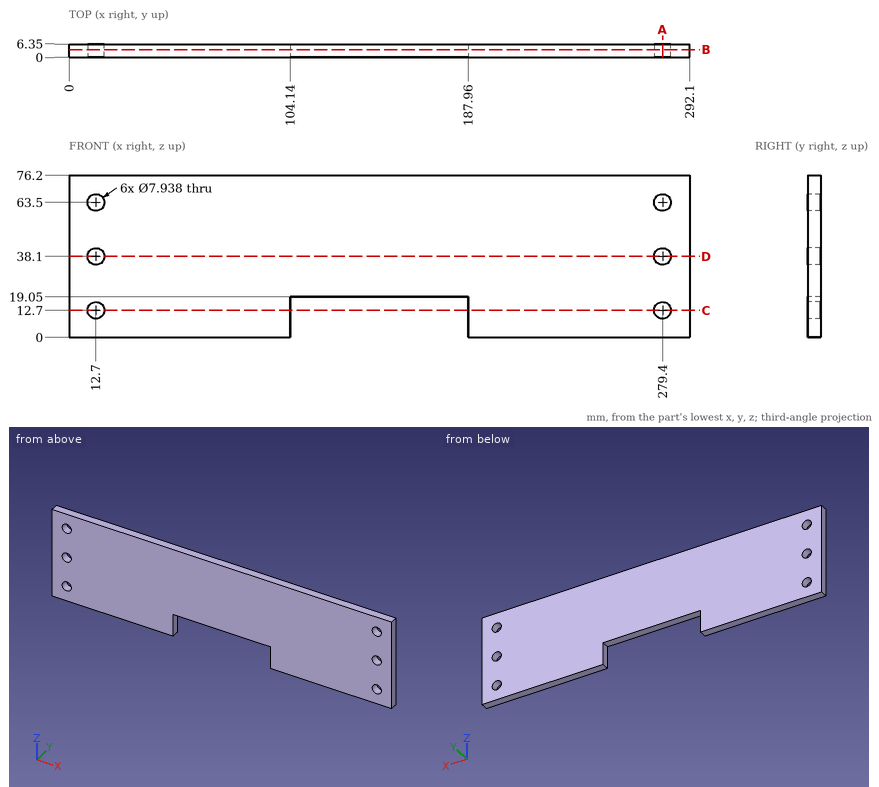
For this review, use the dimensioned drawing (mm, ordinates from the lowest corner) and the shaded views. Round coordinates to 2 decimals unless told otherwise and drop trailing zeros. Write each loop counter-clockwise with the first axis right and the second up, starting at its lowest first coordinate (ties: lowest second). Pieces come first, ordered by that corner, then holes. Notation, with made-up numbers: (73, 33.5) -> (92, 33.5) arc R15 ccw to (92, 61.5) -> close; hole circle Ø8 at (-30, 12.5). An arc over 180 degrees is marked (long way). Answer in a Markdown table with one row per item.
Q1. Take a section at B-B, the plane y = 3.75. State the section outline as (x, z) points.
The answers:
| item | result |
|---|---|
| outline | (0, 0) -> (104.14, 0) -> (104.14, 19.05) -> (187.96, 19.05) -> (187.96, 0) -> (292.1, 0) -> (292.1, 76.2) -> (0, 76.2) -> close; hole circle Ø7.94 at (12.7, 12.7); hole circle Ø7.94 at (12.7, 38.1); hole circle Ø7.94 at (12.7, 63.5); hole circle Ø7.94 at (279.4, 12.7); hole circle Ø7.94 at (279.4, 38.1); hole circle Ø7.94 at (279.4, 63.5) |
Q2. Take a section at C-C, the plane z = 12.7. State the section outline as (x, y) points.
The answers:
| item | result |
|---|---|
| outline | (0, 0) -> (8.73, 0) -> (8.73, 6.35) -> (0, 6.35) -> close; (16.67, 0) -> (104.14, 0) -> (104.14, 6.35) -> (16.67, 6.35) -> close; (187.96, 0) -> (275.43, 0) -> (275.43, 6.35) -> (187.96, 6.35) -> close; (283.37, 0) -> (292.1, 0) -> (292.1, 6.35) -> (283.37, 6.35) -> close |
Q3. Take a section at A-A, the plane x = 279.4. State the section outline as (y, z) points.
The answers:
| item | result |
|---|---|
| outline | (0, 0) -> (6.35, 0) -> (6.35, 8.73) -> (0, 8.73) -> close; (0, 16.67) -> (6.35, 16.67) -> (6.35, 34.13) -> (0, 34.13) -> close; (0, 42.07) -> (6.35, 42.07) -> (6.35, 59.53) -> (0, 59.53) -> close; (0, 67.47) -> (6.35, 67.47) -> (6.35, 76.2) -> (0, 76.2) -> close |
Q4. Clearance check with a flat-ended pin moving along its axis: pin 1 Ø5 at (x, z) = (12.7, 63.5) entering from -Y. State where the tip first meets the part, or that it passes through.
The answers:
| item | result |
|---|---|
| pin 1 | through |
Q5. Take a section at D-D, the plane z = 38.1. State the section outline as (x, y) points, then the cut area to 3 significant figures.
The answers:
| item | result |
|---|---|
| outline | (0, 0) -> (8.73, 0) -> (8.73, 6.35) -> (0, 6.35) -> close; (16.67, 0) -> (275.43, 0) -> (275.43, 6.35) -> (16.67, 6.35) -> close; (283.37, 0) -> (292.1, 0) -> (292.1, 6.35) -> (283.37, 6.35) -> close |
| area | 1,750 mm² |
Q6. To check wall thickness, follow L1, parallel to Z at x = 12.7, y = 2; L2, parallel to X at y = 3.75, z = 38.1; L3, parallel to X at y = 1, z = 4. State the ranges of each line that lie inside material, in increasing order. Write a range as [from, to].
The answers:
| item | result |
|---|---|
| L1 | [0, 8.73], [16.67, 34.13], [42.07, 59.53], [67.47, 76.2] |
| L2 | [0, 8.73], [16.67, 275.43], [283.37, 292.1] |
| L3 | [0, 104.14], [187.96, 292.1] |
